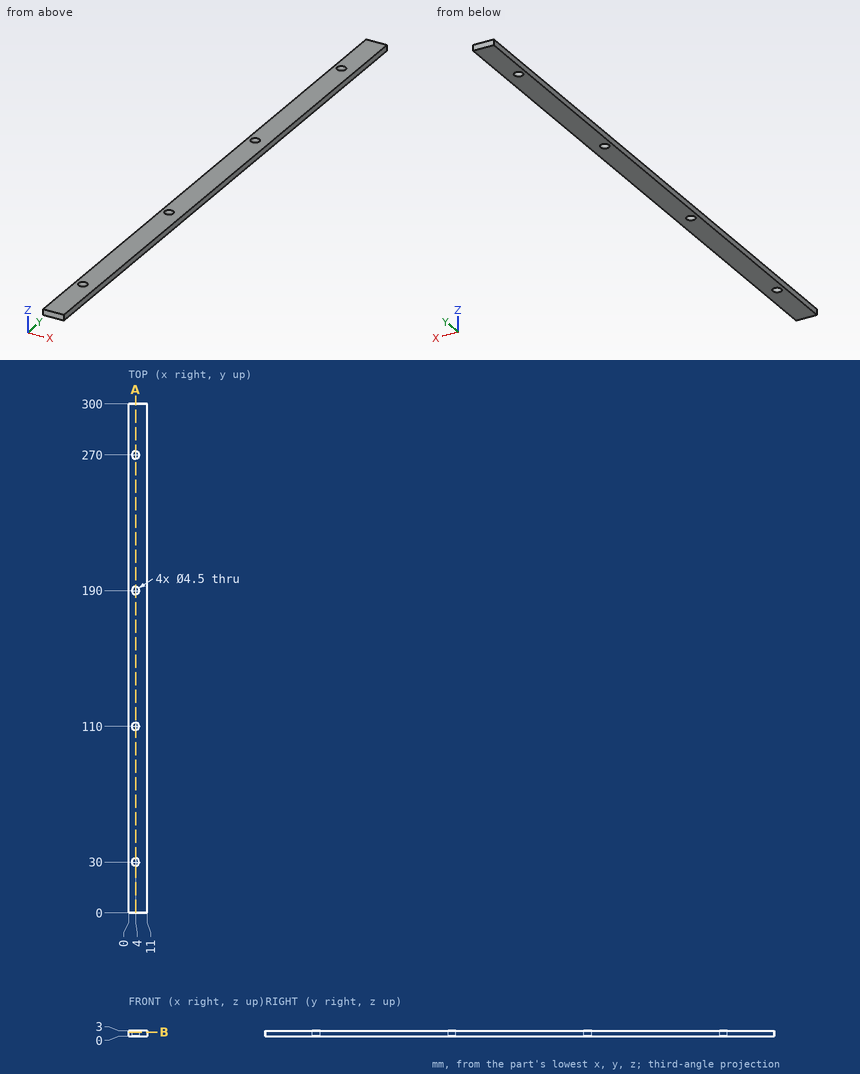
Study the drawing (mm; zero at the part's minimum x, y, z) and answer. Round coordinates to 2 decimals unless told otherwise and drop trailing zeros. Order: outer loops, then holes, each group sorted by start corner. A loop starts at its lowest first (then second) coordinate and runs counter-clockwise, first axis right, second up. Notation, with made-up numbers: (78, 73) - (105, 73) arc R13 ccw to (105, 89) - close; hole circle Ø9 at (-22.5, -34). An arc over 180 degrees is marked (long way). Use one line per item in the form item = value. Start each with the question number.
(1) The part is cut by section A-A (x = 4). Give the vertices of the cut face in (y, z).
(2) Find the intervals of material crossed by line 1 along Y through (x, z) = (4, 1.5); line 2 along X through (y, z) = (190, 1); line 3 along Y through (x, z) = (3, 1), in increasing order. Write a range as from..to.
(3) Flat-ended cylindrical pins translate along their axes: pin 1 Ø6 at (x, y) = (4, 30) entering from +Z; pin 2 Ø4 at (x, y) = (4, 110) entering from -Z. Find the tip coordinate at first contact, or state that the pin passes through.
(4) The part is cut by section B-B (z = 2.25). Give the vertices of the cut face in (x, y), then the cut area to 3 significant figures.
Checked values:
q1.outline = (0, 0) - (27.75, 0) - (27.75, 3) - (0, 3) - close; (32.25, 0) - (107.75, 0) - (107.75, 3) - (32.25, 3) - close; (112.25, 0) - (187.75, 0) - (187.75, 3) - (112.25, 3) - close; (192.25, 0) - (267.75, 0) - (267.75, 3) - (192.25, 3) - close; (272.25, 0) - (300, 0) - (300, 3) - (272.25, 3) - close
q2.line_1 = 0..27.75, 32.25..107.75, 112.25..187.75, 192.25..267.75, 272.25..300
q2.line_2 = 0..1.75, 6.25..11
q2.line_3 = 0..27.98, 32.02..107.98, 112.02..187.98, 192.02..267.98, 272.02..300
q3.pin_1 = 3
q3.pin_2 = through
q4.outline = (0, 0) - (11, 0) - (11, 300) - (0, 300) - close; hole circle Ø4.5 at (4, 30); hole circle Ø4.5 at (4, 110); hole circle Ø4.5 at (4, 190); hole circle Ø4.5 at (4, 270)
q4.area = 3,240 mm^2
